The listing builds one solid part. Answer for the finished solid, in the listing's coordinates (mm). Face numbers are marked on the shaded views. A direction names the side the tool comes from. Give positions to 0.01 mm unless a question says otherwise; leave off trailing zeros. Order: outer loops, then holes, each group sorted by start corner. A loop starts at its lowest first (then second) coordinate and runs counter-clockwise, first axis right, second up. Notation, with made-up numbers: (-36.5, 88) - (5.5, 88) arc R16 ccw to (5.5, 113) - close; hole circle Ø8 at (76.25, 44.5). An arc over 180 degrees is marked (long way). Write each question's results on one line, items separated by ' | '. Start each with the question number.
1. Determine the mould class of the marked faces 4, 5 and 6 for opening direction Z: released by +Z, released by -Z, zero draft, split by the parting line, or undercut.
2. Section D-D (x = 0) is taken. Give the vertices of the cut face in (y, z), and give its area (3 significant figures).
3. Section B-B (z = -9.5) is taken. Give the vertices of the cut face in (x, y).
4. Which of the six approach directions +Z, -Z, +X, -X, +Y, -Y give full straight-line access (tool end or side, diameter ignored) to the marked faces 1, 2 and 3?
5. Flat-ended cylindrical pins translate along their axes: pin 1 (3 mm diameter, centred on x = 0.5, z = 9.5, fed in from -Y); pin 2 (3 mm diameter, centred on x = 1, y = 3, fed in from -Z); pin 3 (2.5 mm diameter, centred on x = 0, y = 1.5, fed in from +Z); pin 4 (2 mm diameter, centred on x = 0, z = 10.5, fed in from +Y). Find the tip coordinate at first contact, or state that the pin passes through.
6. Section A-A (x = 1.5) is taken. Give the vertices of the cut face in (y, z), and give its area (3 significant figures).
7. Section C-C (y = 5.1) is taken. Give the vertices of the cut face in (x, z), and give its area (3 significant figures).
8. Find the intervals of material crossed by L1, parallel to Z at x = -2.75, y = 5.2; L2, parallel to X at y = 5.2, z = -10.5; L3, parallel to X at y = 2.55, z = 0, in increasing order.
from build123d import *

# Parameters (mm, degrees)
SKETCH1_W           = 8.763
SKETCH1_H           = 8.763
SKETCH1_W_2         = 5.763
SKETCH1_H_2         = 5.763
BOSS_EXTRUDE1_DEPTH = 1.2
SKETCH2_W           = 13
SKETCH2_H           = 13
SKETCH2_W_2         = 8.763
SKETCH2_H_2         = 8.763
BOSS_EXTRUDE3_DEPTH = 5.9
CHAMFER1_SIZE       = 1.5
SKETCH3_W           = 13
SKETCH3_H           = 6
SKETCH3_R           = 1.25
BOSS_EXTRUDE4_DEPTH = 1.2
BOSS_EXTRUDE5_DEPTH = 2
FILLET1_R           = 1
CUT_EXTRUDE1_REACH  = 20.975
SKETCH4_W           = 8.763
SKETCH4_H           = 3


with BuildPart() as part:
    # Sketch1 → Boss-Extrude1 (new body)
    with BuildSketch(Plane(origin=(0, 0, 0), x_dir=(1, 0, 0), z_dir=(0, 1, 0))):
        Rectangle(SKETCH1_W, SKETCH1_H)
        Rectangle(SKETCH1_W_2, SKETCH1_H_2, mode=Mode.SUBTRACT)
    extrude(amount=BOSS_EXTRUDE1_DEPTH)

    # Sketch2 → Boss-Extrude3 (add)
    with BuildSketch(Plane.XZ):
        Rectangle(SKETCH2_W, SKETCH2_H)
        Rectangle(SKETCH2_W_2, SKETCH2_H_2, mode=Mode.SUBTRACT)
    extrude(amount=-BOSS_EXTRUDE3_DEPTH)

    # Chamfer1
    # the kernel refuses this chamfer: 1.5 mm, written as the material it takes off along each edge
    with BuildSketch(Plane(origin=(2.8815, 1.2, -2.8815), x_dir=(0, 0.02749587661058634, -0.9996219169112968), z_dir=(-1, 0, 0))) as chamfer1_piece_1_section:
        Polygon((CHAMFER1_SIZE * 0.999621916911, CHAMFER1_SIZE * 0.0274958766106), (-CHAMFER1_SIZE * 0.0274958766106, CHAMFER1_SIZE * 0.999621916911), (0, 0), align=None)
    chamfer1_piece_1 = extrude(amount=5.763, mode=Mode.PRIVATE)
    chamfer1_piece_1 = split(chamfer1_piece_1, bisect_by=Plane(origin=(0, 0.704393769, -4.3815), z_dir=(0, 0, 1)), keep=Keep.TOP, mode=Mode.PRIVATE)
    add(chamfer1_piece_1, mode=Mode.SUBTRACT)
    with BuildSketch(Plane(origin=(2.8815, 1.2, 2.8815), x_dir=(-0.02749587661058649, -0.9996219169112968, 0), z_dir=(0, 0, -1))) as chamfer1_piece_2_section:
        Polygon((CHAMFER1_SIZE * 0.999621916911, -CHAMFER1_SIZE * 0.0274958766106), (-CHAMFER1_SIZE * 0.0274958766106, -CHAMFER1_SIZE * 0.999621916911), (0, 0), align=None)
    chamfer1_piece_2 = extrude(amount=5.763, mode=Mode.PRIVATE)
    chamfer1_piece_2 = split(chamfer1_piece_2, bisect_by=Plane(origin=(4.3815, 0.704393769, 0), z_dir=(-1, 0, 0)), keep=Keep.TOP, mode=Mode.PRIVATE)
    add(chamfer1_piece_2, mode=Mode.SUBTRACT)
    with BuildSketch(Plane(origin=(-2.8815, 1.2, 2.8815), x_dir=(0, -0.9996219169112968, -0.02749587661058649), z_dir=(1, 0, 0))) as chamfer1_piece_3_section:
        Polygon((CHAMFER1_SIZE * 0.999621916911, -CHAMFER1_SIZE * 0.0274958766106), (-CHAMFER1_SIZE * 0.0274958766106, -CHAMFER1_SIZE * 0.999621916911), (0, 0), align=None)
    chamfer1_piece_3 = extrude(amount=5.763, mode=Mode.PRIVATE)
    chamfer1_piece_3 = split(chamfer1_piece_3, bisect_by=Plane(origin=(0, 0.704393769, 4.3815), z_dir=(0, 0, -1)), keep=Keep.TOP, mode=Mode.PRIVATE)
    add(chamfer1_piece_3, mode=Mode.SUBTRACT)
    with BuildSketch(Plane(origin=(-2.8815, 1.2, -2.8815), x_dir=(0.02749587661058649, -0.9996219169112968, 0), z_dir=(0, 0, 1))) as chamfer1_piece_4_section:
        Polygon((CHAMFER1_SIZE * 0.999621916911, -CHAMFER1_SIZE * 0.0274958766106), (-CHAMFER1_SIZE * 0.0274958766106, -CHAMFER1_SIZE * 0.999621916911), (0, 0), align=None)
    chamfer1_piece_4 = extrude(amount=5.763, mode=Mode.PRIVATE)
    chamfer1_piece_4 = split(chamfer1_piece_4, bisect_by=Plane(origin=(-4.3815, 0.704393769, 0), z_dir=(1, 0, 0)), keep=Keep.TOP, mode=Mode.PRIVATE)
    add(chamfer1_piece_4, mode=Mode.SUBTRACT)
    with BuildSketch(Plane(origin=(2.8815, 1.2, 2.8815), x_dir=(-0.02749587661058649, -0.9996219169112968, 0), z_dir=(0, 0, -1))) as chamfer1_piece_5a_section:
        Polygon((CHAMFER1_SIZE * 0.999621916911, -CHAMFER1_SIZE * 0.0274958766106), (-CHAMFER1_SIZE * 0.0274958766106, -CHAMFER1_SIZE * 0.999621916911), (0, 0), align=None)
    chamfer1_piece_5a = extrude(amount=9.620524482, mode=Mode.PRIVATE)
    chamfer1_piece_5a = split(chamfer1_piece_5a, bisect_by=Plane(origin=(3.374451501, 0.704393769, -2.8815), z_dir=(0, 0, -1)), keep=Keep.TOP, mode=Mode.PRIVATE)
    chamfer1_piece_5a = split(chamfer1_piece_5a, bisect_by=Plane(origin=(3.374451501, 0.704393769, -4.3815), z_dir=(0, 0, 1)), keep=Keep.TOP, mode=Mode.PRIVATE)
    chamfer1_piece_5a = split(chamfer1_piece_5a, bisect_by=Plane(origin=(4.3815, 0.704393769, -3.6315), z_dir=(-1, 0, 0)), keep=Keep.TOP, mode=Mode.PRIVATE)
    with BuildSketch(Plane(origin=(6.739024482, 1.2, -2.8815), x_dir=(0, 0.02749587661058634, -0.9996219169112968), z_dir=(-1, 0, 0))) as chamfer1_piece_5b_section:
        Polygon((CHAMFER1_SIZE * 0.999621916911, CHAMFER1_SIZE * 0.0274958766106), (-CHAMFER1_SIZE * 0.0274958766106, CHAMFER1_SIZE * 0.999621916911), (0, 0), align=None)
    chamfer1_piece_5b = extrude(amount=9.620524482, mode=Mode.PRIVATE)
    chamfer1_piece_5b = split(chamfer1_piece_5b, bisect_by=Plane(origin=(2.8815, 0.704393769, -3.374451501), z_dir=(1, 0, 0)), keep=Keep.TOP, mode=Mode.PRIVATE)
    chamfer1_piece_5b = split(chamfer1_piece_5b, bisect_by=Plane(origin=(3.6315, 0.704393769, -4.3815), z_dir=(0, 0, 1)), keep=Keep.TOP, mode=Mode.PRIVATE)
    chamfer1_piece_5b = split(chamfer1_piece_5b, bisect_by=Plane(origin=(4.3815, 0.704393769, -3.374451501), z_dir=(-1, 0, 0)), keep=Keep.TOP, mode=Mode.PRIVATE)
    chamfer1_piece_5 = chamfer1_piece_5a & chamfer1_piece_5b
    add(chamfer1_piece_5, mode=Mode.SUBTRACT)
    with BuildSketch(Plane(origin=(-2.8815, 1.2, -6.739024482), x_dir=(0.02749587661058649, -0.9996219169112968, 0), z_dir=(0, 0, 1))) as chamfer1_piece_6a_section:
        Polygon((CHAMFER1_SIZE * 0.999621916911, -CHAMFER1_SIZE * 0.0274958766106), (-CHAMFER1_SIZE * 0.0274958766106, -CHAMFER1_SIZE * 0.999621916911), (0, 0), align=None)
    chamfer1_piece_6a = extrude(amount=9.620524482, mode=Mode.PRIVATE)
    chamfer1_piece_6a = split(chamfer1_piece_6a, bisect_by=Plane(origin=(-3.374451501, 0.704393769, -2.8815), z_dir=(0, 0, -1)), keep=Keep.TOP, mode=Mode.PRIVATE)
    chamfer1_piece_6a = split(chamfer1_piece_6a, bisect_by=Plane(origin=(-3.374451501, 0.704393769, -4.3815), z_dir=(0, 0, 1)), keep=Keep.TOP, mode=Mode.PRIVATE)
    chamfer1_piece_6a = split(chamfer1_piece_6a, bisect_by=Plane(origin=(-4.3815, 0.704393769, -3.6315), z_dir=(1, 0, 0)), keep=Keep.TOP, mode=Mode.PRIVATE)
    with BuildSketch(Plane(origin=(2.8815, 1.2, -2.8815), x_dir=(0, 0.02749587661058634, -0.9996219169112968), z_dir=(-1, 0, 0))) as chamfer1_piece_6b_section:
        Polygon((CHAMFER1_SIZE * 0.999621916911, CHAMFER1_SIZE * 0.0274958766106), (-CHAMFER1_SIZE * 0.0274958766106, CHAMFER1_SIZE * 0.999621916911), (0, 0), align=None)
    chamfer1_piece_6b = extrude(amount=9.620524482, mode=Mode.PRIVATE)
    chamfer1_piece_6b = split(chamfer1_piece_6b, bisect_by=Plane(origin=(-2.8815, 0.704393769, -3.374451501), z_dir=(-1, 0, 0)), keep=Keep.TOP, mode=Mode.PRIVATE)
    chamfer1_piece_6b = split(chamfer1_piece_6b, bisect_by=Plane(origin=(-3.6315, 0.704393769, -4.3815), z_dir=(0, 0, 1)), keep=Keep.TOP, mode=Mode.PRIVATE)
    chamfer1_piece_6b = split(chamfer1_piece_6b, bisect_by=Plane(origin=(-4.3815, 0.704393769, -3.374451501), z_dir=(1, 0, 0)), keep=Keep.TOP, mode=Mode.PRIVATE)
    chamfer1_piece_6 = chamfer1_piece_6a & chamfer1_piece_6b
    add(chamfer1_piece_6, mode=Mode.SUBTRACT)
    with BuildSketch(Plane(origin=(-2.8815, 1.2, 2.8815), x_dir=(0, -0.9996219169112968, -0.02749587661058649), z_dir=(1, 0, 0))) as chamfer1_piece_7a_section:
        Polygon((CHAMFER1_SIZE * 0.999621916911, -CHAMFER1_SIZE * 0.0274958766106), (-CHAMFER1_SIZE * 0.0274958766106, -CHAMFER1_SIZE * 0.999621916911), (0, 0), align=None)
    chamfer1_piece_7a = extrude(amount=9.620524482, mode=Mode.PRIVATE)
    chamfer1_piece_7a = split(chamfer1_piece_7a, bisect_by=Plane(origin=(2.8815, 0.704393769, 3.374451501), z_dir=(1, 0, 0)), keep=Keep.TOP, mode=Mode.PRIVATE)
    chamfer1_piece_7a = split(chamfer1_piece_7a, bisect_by=Plane(origin=(4.3815, 0.704393769, 3.374451501), z_dir=(-1, 0, 0)), keep=Keep.TOP, mode=Mode.PRIVATE)
    chamfer1_piece_7a = split(chamfer1_piece_7a, bisect_by=Plane(origin=(3.6315, 0.704393769, 4.3815), z_dir=(0, 0, -1)), keep=Keep.TOP, mode=Mode.PRIVATE)
    with BuildSketch(Plane(origin=(2.8815, 1.2, 6.739024482), x_dir=(-0.02749587661058649, -0.9996219169112968, 0), z_dir=(0, 0, -1))) as chamfer1_piece_7b_section:
        Polygon((CHAMFER1_SIZE * 0.999621916911, -CHAMFER1_SIZE * 0.0274958766106), (-CHAMFER1_SIZE * 0.0274958766106, -CHAMFER1_SIZE * 0.999621916911), (0, 0), align=None)
    chamfer1_piece_7b = extrude(amount=9.620524482, mode=Mode.PRIVATE)
    chamfer1_piece_7b = split(chamfer1_piece_7b, bisect_by=Plane(origin=(3.374451501, 0.704393769, 2.8815), z_dir=(0, 0, 1)), keep=Keep.TOP, mode=Mode.PRIVATE)
    chamfer1_piece_7b = split(chamfer1_piece_7b, bisect_by=Plane(origin=(4.3815, 0.704393769, 3.6315), z_dir=(-1, 0, 0)), keep=Keep.TOP, mode=Mode.PRIVATE)
    chamfer1_piece_7b = split(chamfer1_piece_7b, bisect_by=Plane(origin=(3.374451501, 0.704393769, 4.3815), z_dir=(0, 0, -1)), keep=Keep.TOP, mode=Mode.PRIVATE)
    chamfer1_piece_7 = chamfer1_piece_7a & chamfer1_piece_7b
    add(chamfer1_piece_7, mode=Mode.SUBTRACT)
    with BuildSketch(Plane(origin=(-6.739024482, 1.2, 2.8815), x_dir=(0, -0.9996219169112968, -0.02749587661058649), z_dir=(1, 0, 0))) as chamfer1_piece_8a_section:
        Polygon((CHAMFER1_SIZE * 0.999621916911, -CHAMFER1_SIZE * 0.0274958766106), (-CHAMFER1_SIZE * 0.0274958766106, -CHAMFER1_SIZE * 0.999621916911), (0, 0), align=None)
    chamfer1_piece_8a = extrude(amount=9.620524482, mode=Mode.PRIVATE)
    chamfer1_piece_8a = split(chamfer1_piece_8a, bisect_by=Plane(origin=(-2.8815, 0.704393769, 3.374451501), z_dir=(-1, 0, 0)), keep=Keep.TOP, mode=Mode.PRIVATE)
    chamfer1_piece_8a = split(chamfer1_piece_8a, bisect_by=Plane(origin=(-3.6315, 0.704393769, 4.3815), z_dir=(0, 0, -1)), keep=Keep.TOP, mode=Mode.PRIVATE)
    chamfer1_piece_8a = split(chamfer1_piece_8a, bisect_by=Plane(origin=(-4.3815, 0.704393769, 3.374451501), z_dir=(1, 0, 0)), keep=Keep.TOP, mode=Mode.PRIVATE)
    with BuildSketch(Plane(origin=(-2.8815, 1.2, -2.8815), x_dir=(0.02749587661058649, -0.9996219169112968, 0), z_dir=(0, 0, 1))) as chamfer1_piece_8b_section:
        Polygon((CHAMFER1_SIZE * 0.999621916911, -CHAMFER1_SIZE * 0.0274958766106), (-CHAMFER1_SIZE * 0.0274958766106, -CHAMFER1_SIZE * 0.999621916911), (0, 0), align=None)
    chamfer1_piece_8b = extrude(amount=9.620524482, mode=Mode.PRIVATE)
    chamfer1_piece_8b = split(chamfer1_piece_8b, bisect_by=Plane(origin=(-3.374451501, 0.704393769, 2.8815), z_dir=(0, 0, 1)), keep=Keep.TOP, mode=Mode.PRIVATE)
    chamfer1_piece_8b = split(chamfer1_piece_8b, bisect_by=Plane(origin=(-3.374451501, 0.704393769, 4.3815), z_dir=(0, 0, -1)), keep=Keep.TOP, mode=Mode.PRIVATE)
    chamfer1_piece_8b = split(chamfer1_piece_8b, bisect_by=Plane(origin=(-4.3815, 0.704393769, 3.6315), z_dir=(1, 0, 0)), keep=Keep.TOP, mode=Mode.PRIVATE)
    chamfer1_piece_8 = chamfer1_piece_8a & chamfer1_piece_8b
    add(chamfer1_piece_8, mode=Mode.SUBTRACT)

    # Sketch3 → Boss-Extrude4 (add)
    with BuildSketch(Plane(origin=(0, 5.9, 0), x_dir=(1, 0, 0), z_dir=(0, 1, 0))):
        with Locations((0, 9.5)):
            Rectangle(SKETCH3_W, SKETCH3_H)
        with Locations(Location((0, 10.5, 0), (0, 0, 270))):
            Circle(SKETCH3_R, mode=Mode.SUBTRACT)
    boss_extrude4 = extrude(amount=-BOSS_EXTRUDE4_DEPTH)

    # Mirror1: Boss-Extrude4 across plane
    add(boss_extrude4.mirror(Plane.XY))

    # Sketch5 → Boss-Extrude5 (add)
    with BuildSketch(Plane.ZY.offset(6.5)):
        Polygon((6.5, 4.7), (6.5, 0), (12.5, 4.7), align=None)
        Polygon((-6.5, 4.7), (-6.5, 0), (-12.5, 4.7), align=None)
    boss_extrude5 = extrude(amount=-BOSS_EXTRUDE5_DEPTH)

    # Mirror2: Boss-Extrude5 across plane
    add(boss_extrude5.mirror(Plane(origin=(0, 0, 0), x_dir=(0, 0, 1), z_dir=(1, 0, 0))))

    # Fillet1
    fillet1_edges = [part.edges().sort_by_distance(p)[0] for p in [
        (-4.5, 2.35, -6.5),
        (4.5, 2.35, 6.5),
        (4.5, 2.35, -6.5),
        (-6.5, 5.3, -12.5),
        (6.5, 5.3, -12.5),
        (-6.5, 5.3, 12.5),
        (6.5, 5.3, 12.5),
        (-4.5, 2.35, 6.5),
    ]]
    fillet(fillet1_edges, radius=FILLET1_R)

    # Sketch4 → Cut-Extrude1 (cut, up to next)
    with BuildSketch(Plane.ZY.offset(6.5), mode=Mode.PRIVATE) as cut_extrude1_sk1:
        with Locations((0, 4.4)):
            Rectangle(SKETCH4_W, SKETCH4_H)
    cut_extrude1_tool1 = extrude(cut_extrude1_sk1.sketch, amount=-CUT_EXTRUDE1_REACH, mode=Mode.PRIVATE) & part.part
    add(cut_extrude1_tool1.solids().sort_by_distance((-6.5, 4.4, 0))[0], mode=Mode.SUBTRACT)


solid = part.part
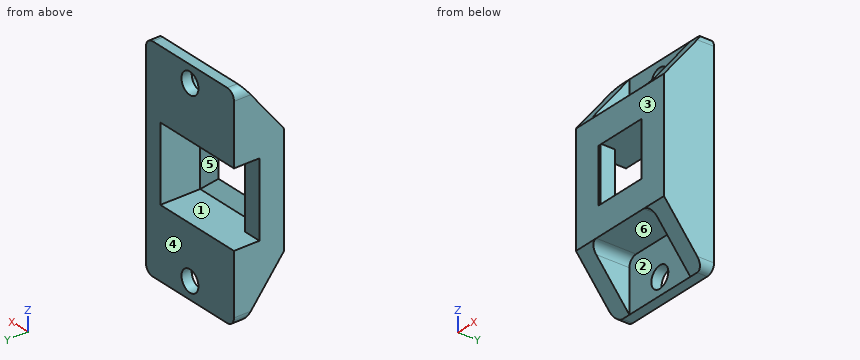
Reported:
1) face 4: zero draft | face 5: undercut | face 6: released by -Z
2) outline: (0, -6.5) - (4.7, -6.5) - (4.7, -9.25) - (5.9, -9.25) - (5.9, -4.38) - (1.2, -4.38) - (0, -3.18) - close; (0, 3.18) - (1.2, 4.38) - (5.9, 4.38) - (5.9, 9.25) - (4.7, 9.25) - (4.7, 6.5) - (0, 6.5) - close; (4.7, -12.5) - (5.9, -12.5) - (5.9, -11.75) - (4.7, -11.75) - close; (4.7, 11.75) - (5.9, 11.75) - (5.9, 12.5) - (4.7, 12.5) - close | area: 34.8 mm²
3) outline: (-6.5, 2.35) - (-4.5, 2.35) - (-4.5, 4.7) - (-0.75, 4.7) - (-0.75, 5.9) - (-6.5, 5.9) - close; (0.75, 4.7) - (4.5, 4.7) - (4.5, 2.35) - (6.5, 2.35) - (6.5, 5.9) - (0.75, 5.9) - close
4) face 1: +Y | face 2: -Z, -Y | face 3: +Z, -Z, +X, -X, -Y
5) pin 1: y = 4.7 | pin 2: z = -6.5 | pin 3: z = 6.5 | pin 4: through
6) outline: (0, -6.5) - (4.7, -6.5) - (4.7, -12.5) - (5.9, -12.5) - (5.9, -4.38) - (1.2, -4.38) - (0, -3.18) - close; (0, 3.18) - (1.2, 4.38) - (5.9, 4.38) - (5.9, 12.5) - (4.7, 12.5) - (4.7, 6.5) - (0, 6.5) - close | area: 40.8 mm²
7) outline: (-6.5, -11.5) arc R1 ccw to (-5.5, -12.5) - (5.5, -12.5) arc R1 ccw to (6.5, -11.5) - (6.5, 11.5) arc R1 ccw to (5.5, 12.5) - (-5.5, 12.5) arc R1 ccw to (-6.5, 11.5) - (-6.5, 4.38) - (4.38, 4.38) - (4.38, -4.38) - (-6.5, -4.38) - close; hole circle Ø2.5 at (0, -10.5); hole circle Ø2.5 at (0, 10.5) | area: 219 mm²
8) L1: -12.5 to -4.38, 4.38 to 12.5 | L2: -6.5 to -1.25, 1.25 to 6.5 | L3: -6.5 to -4.38, 4.38 to 6.5
